Read the model definition and answer for the solid it produces. Units are mm, in the model's axes. Coordinates: 2 decimals unless noted, no trailing zeros. Order: outer loops, then holes, each group sorted by start corner. A loop starts at its lowest first (then second) coordinate and runs counter-clockwise, first axis right, second up. Notation, with made-up numbers: M 35,63 L 85,63 A22 cw 85,90 Z; hole C 50.25,37.25 d1. An arc over 180 degrees is marked long. Use a Markdown table: item, result. Add a question column.
1) This flat-tipped pin is pushed along its axis until it touches: pin 1 Ø1 at (x, z) = (16, 1.5) entering from +Y. Where does it stop, or does it pass through?
2) Find section A-A on x = 64. Write down the section's boundary in (y, z).
3) Find the intervals of material crossed by probe 1 along Z at (x, y) = (-46.5, 1.35); probe 2 along Y at (x, z) = (31.5, 0.1); probe 3 along Y at (x, z) = (73.5, 1.3), in increasing order. Write a range as [from, to].
Solid Edge part; units mm, degrees
sketch "Sketch1" plane through (0, 0, 0) normal (1, 0, 0) x (0, 1, 0)
  circle A0 centre (0, 0) radius 2
extrude "Protrusion1" add sketch "Sketch1" along normal mid plane 160
cosmetic_thread "Thread_3" thread depth 8
cosmetic_thread "Thread_4" thread depth 8
chamfer "Chamfer_1" distance 0.5 angle 45 1 edges at (-80, -2, 0) measured on face at (-80, 1.2933, -1.3733)
chamfer "Chamfer_2" distance 0.5 angle 45 1 edges at (80, -2, 0) measured on face at (80, 1.2933, -1.3733)
Check result:
| question | item | result |
|---|---|---|
| 1 | pin 1 | stops at y = 1.73 |
| 2 | outline | C 0,0 d4 |
| 3 | probe 1 | z = [-1.48, 1.48] |
| 3 | probe 2 | y = [-2, 2] |
| 3 | probe 3 | y = [-1.52, 1.52] |
